Read the model definition and answer for the solid it produces. Units are mm, in the model's axes. Coordinates: 2 decimals unless noted, no trailing zeros. Loops run counter-clockwise (first coordinate to the right, second up) from the corner with the lowest first, then second, coordinate; pieces in that order, holes last.
from build123d import *

# Parameters (mm, degrees)
SKETCH2_W           = 75
SKETCH2_H           = 75
SKETCH2_R           = 15.119722523
SKETCH2_R_2         = 1
SKETCH2_R_3         = 4
SKETCH2_W_2         = 10
SKETCH2_H_2         = 2.5
BOSS_EXTRUDE2_DEPTH = 5
FILLET1_R           = 8


with BuildPart() as part:
    # Sketch2 → Boss-Extrude2 (new body)
    with BuildSketch(Plane(origin=(0, 0, 0), x_dir=(1, 0, 0), z_dir=(0, 1, 0))):
        Rectangle(SKETCH2_W, SKETCH2_H)
        with Locations(Location((0, 0, 0), (0, 0, 270))):
            Circle(SKETCH2_R, mode=Mode.SUBTRACT)
        with Locations(Location((-23, 0, 0), (0, 0, 270))):
            Circle(SKETCH2_R_2, mode=Mode.SUBTRACT)
        with Locations(Location((23, 0, 0), (0, 0, 90))):
            Circle(SKETCH2_R_2, mode=Mode.SUBTRACT)
        with Locations(Location((29.242640687, 20.757359313, 0), (0, 0, 270))):
            Circle(SKETCH2_R_3, mode=Mode.SUBTRACT)
        with Locations(Location((20.757359313, 29.242640687, 0), (0, 0, 90))):
            Circle(SKETCH2_R_3, mode=Mode.SUBTRACT)
        with Locations(Location((-20.757359313, -29.242640687, 0), (0, 0, 90))):
            Circle(SKETCH2_R_3, mode=Mode.SUBTRACT)
        with Locations(Location((-29.242640687, -20.757359313, 0), (0, 0, 270))):
            Circle(SKETCH2_R_3, mode=Mode.SUBTRACT)
        with Locations(Location((-20.757359313, 29.242640687, 0), (0, 0, 270))):
            Circle(SKETCH2_R_3, mode=Mode.SUBTRACT)
        with Locations(Location((-29.242640687, 20.757359313, 0), (0, 0, 90))):
            Circle(SKETCH2_R_3, mode=Mode.SUBTRACT)
        with Locations(Location((29.242640687, -20.757359313, 0), (0, 0, 90))):
            Circle(SKETCH2_R_3, mode=Mode.SUBTRACT)
        with Locations(Location((20.757359313, -29.242640687, 0), (0, 0, 270))):
            Circle(SKETCH2_R_3, mode=Mode.SUBTRACT)
        with Locations((0, -23.559960871)):
            Rectangle(SKETCH2_W_2, SKETCH2_H_2, mode=Mode.SUBTRACT)
        with Locations((0, 23.559960871)):
            Rectangle(SKETCH2_W_2, SKETCH2_H_2, mode=Mode.SUBTRACT)
    extrude(amount=BOSS_EXTRUDE2_DEPTH)

    # Fillet1
    fillet1_edges = [part.edges().sort_by_distance(p)[0] for p in [
        (37.5, 2.5, 37.5),
        (-37.5, 2.5, 37.5),
        (-37.5, 2.5, -37.5),
        (37.5, 2.5, -37.5),
    ]]
    fillet(fillet1_edges, radius=FILLET1_R)


solid = part.part
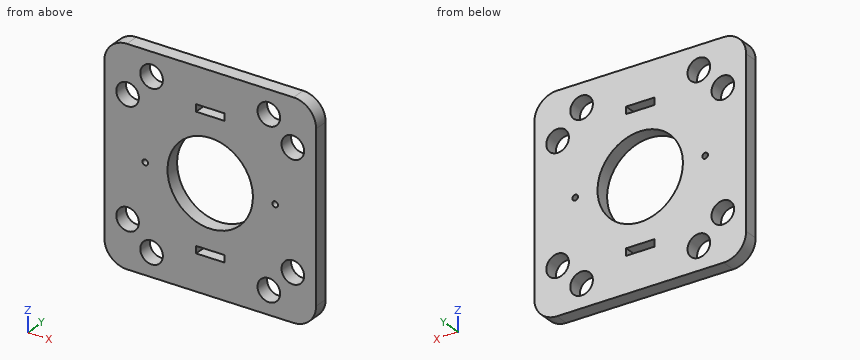
Q1. A cutting plane is placed at D-D (z = -23.5). Give the vertices of the cut face in (x, y), then the cut area to 3 significant figures.
Findings below:
outline: (-37.5, 0) - (-32.15, 0) - (-32.15, 5) - (-37.5, 5) - close; (-26.33, 0) - (-5, 0) - (-5, 5) - (-26.33, 5) - close; (5, 0) - (26.33, 0) - (26.33, 5) - (5, 5) - close; (32.15, 0) - (37.5, 0) - (37.5, 5) - (32.15, 5) - close
area: 267 mm2
Q2. A cutting plane is placed at C-C (y = 0.75). Count the separate pieces of the cut face and the enclosed holes in it, then the cut area to 3 significant figures.
Findings below:
separate pieces: 1
enclosed holes: 13
area: 4,390 mm2
Q3. A cutting plane is placed at A-A (x = 0). Give the vertices of the cut face in (y, z).
Findings below:
outline: (0, -37.5) - (5, -37.5) - (5, -24.81) - (0, -24.81) - close; (0, -22.31) - (5, -22.31) - (5, -15.12) - (0, -15.12) - close; (0, 15.12) - (5, 15.12) - (5, 22.31) - (0, 22.31) - close; (0, 24.81) - (5, 24.81) - (5, 37.5) - (0, 37.5) - close
Q4. Straight lines are drawn through the part: probe 1 along X at (y, z) = (1.35, 0); probe 2 along Z at (x, y) = (-21, 0.55). For each, find the intervals that lie inside material, in ascending order.
Findings below:
probe 1: x = -37.5 to -24, -22 to -15.12, 15.12 to 22, 24 to 37.5
probe 2: z = -37.5 to -33.24, -25.25 to 25.25, 33.24 to 37.5
Q5. A cutting plane is placed at B-B (z = 9). Give the vertices of the cut face in (x, y), then the cut area to 3 significant figures.
Findings below:
outline: (-37.5, 0) - (-12.15, 0) - (-12.15, 5) - (-37.5, 5) - close; (12.15, 0) - (37.5, 0) - (37.5, 5) - (12.15, 5) - close
area: 254 mm2
